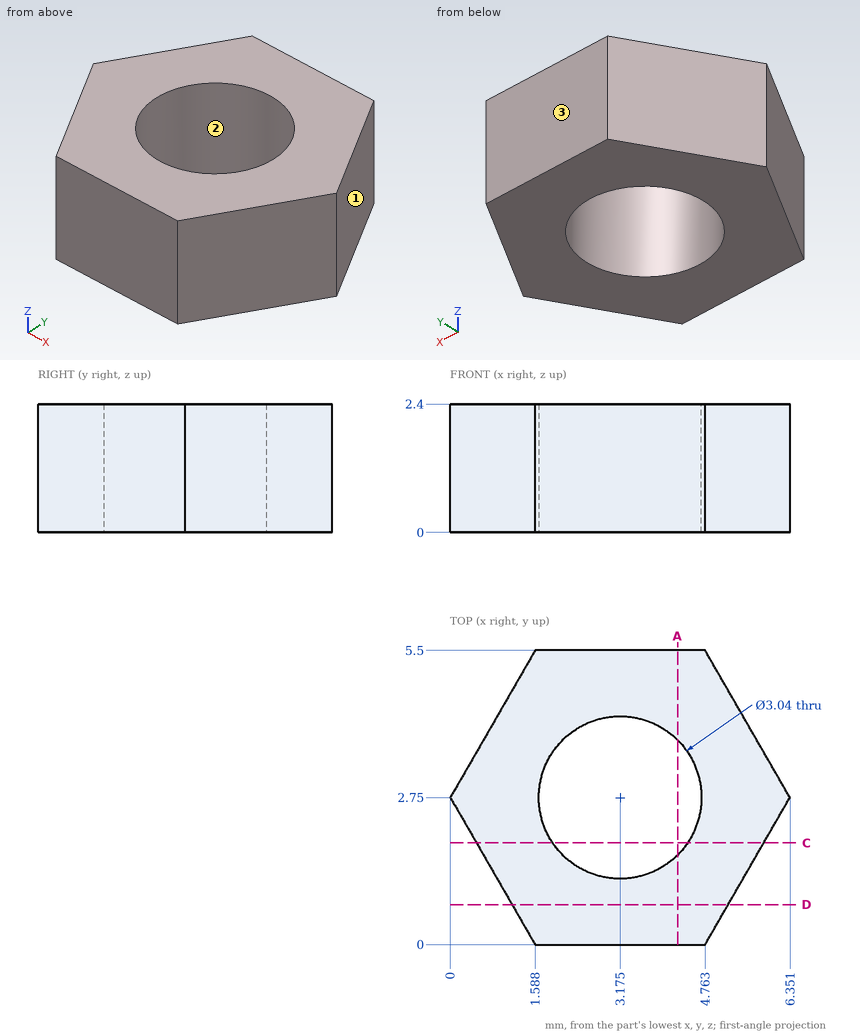
Drawing for the job (mm, zero at the part's lowest x, y, z). Give positions to 0.01 mm unless a question says otherwise; leave off trailing zeros. Order: outer loops, then holes, each group sorted by start corner. A loop starts at its lowest first (then second) coordinate and runs counter-clockwise, first axis right, second up. Notation, with made-up numbers: M -17,75 L -12,75 A28 cw -12,100 Z; hole C 67,85.25 d11. An arc over 180 degrees is marked long. Write item = value, one per line. Start each with the question number.
(1) Slice it at C-C on y = 1.9. Write the cut outline in (x, z) (1 decimal).
(2) Slice it at D-D on y = 0.75. Write the cut outline in (x, z) (1 decimal).
(3) Probe L1, parallel to X at y = 1.65, z = 2.35 (1 decimal); L2, parallel to Y at x = 3, z = 1.1; L3, parallel to Y at x = 2.5, z = 0.8. List the from-to ranges inside material, lowest first. Write a range as [from, to].
(4) Two-plate mould, pull along X, no slides. Class the marked faces 1, 2 and 3: released by +X, released by -X, zero draft, split by the parting line, or undercut.
(5) Pin check, flat tips, straight feed: pin 1 Ø1.8 at (x, y) = (3.18, 2.75) entering from -Z; pin 2 Ø1 at (y, z) = (3.5, 0.5) entering from -X (1 decimal). Stop position of each tip, or through.
(6) Slice it at A-A on x = 4.25. Write the cut outline in (y, z) (1 decimal).
Responses:
q1.outline = M 0.5,0 L 1.9,0 L 1.9,2.4 L 0.5,2.4 Z; M 4.4,0 L 5.9,0 L 5.9,2.4 L 4.4,2.4 Z
q2.outline = M 1.2,0 L 5.2,0 L 5.2,2.4 L 1.2,2.4 Z
q3.L1 = [0.6, 2.1], [4.2, 5.7]
q3.L2 = [0, 1.24], [4.26, 5.5]
q3.L3 = [0, 1.39], [4.11, 5.5]
q4.face_1 = released by +X
q4.face_2 = undercut
q4.face_3 = zero draft
q5.pin_1 = through
q5.pin_2 = 0.1
q6.outline = M 0,0 L 1.7,0 L 1.7,2.4 L 0,2.4 Z; M 3.8,0 L 5.5,0 L 5.5,2.4 L 3.8,2.4 Z
